```python
from build123d import *

# Parameters (mm, degrees)
SKETCH1_W             = 66.675
SKETCH1_H             = 234.95
BOSS_EXTRUDE1_DEPTH   = 3.175
SKETCH3_W             = 12.7
SKETCH3_H             = 3.175
BOSS_EXTRUDE2_DEPTH   = 3.175
CUT_EXTRUDE1_DEPTH    = 126.211389383
FILLET1_R             = 0.508
F_6_32_TAPPED_HOLE1_D = 2.7051


with BuildPart() as part:
    # Sketch1 → Boss-Extrude1 (new body)
    with BuildSketch(Plane(origin=(0, 0, 0), x_dir=(1, 0, 0), z_dir=(0, 1, 0))):
        Rectangle(SKETCH1_W, SKETCH1_H)
    extrude(amount=BOSS_EXTRUDE1_DEPTH)

    # Sketch3 → Boss-Extrude2 (add)
    with BuildSketch(Plane(origin=(0, 3.175, 0), x_dir=(1, 0, 0), z_dir=(0, 1, 0))):
        with Locations((-19.05, -119.0625)):
            Rectangle(SKETCH3_W, SKETCH3_H)
        with Locations((19.05, -119.0625)):
            Rectangle(SKETCH3_W, SKETCH3_H)
        with Locations((19.05, 119.0625)):
            Rectangle(SKETCH3_W, SKETCH3_H)
        with Locations((-19.05, 119.0625)):
            Rectangle(SKETCH3_W, SKETCH3_H)
    extrude(amount=-BOSS_EXTRUDE2_DEPTH)

    # Sketch4 → Cut-Extrude1 (cut, through all)
    with BuildSketch(Plane(origin=(0, 3.175, 0), x_dir=(1, 0, 0), z_dir=(0, 1, 0))):
        with BuildLine():
            Line((-12.7, 111.125), (12.7, 111.125))
            ThreePointArc((12.7, 111.125), (19.05, 104.775), (12.7, 98.425))
            Line((12.7, 98.425), (-12.7, 98.425))
            ThreePointArc((-12.7, 98.425), (-19.05, 104.775), (-12.7, 111.125))
        make_face()
    extrude(amount=-CUT_EXTRUDE1_DEPTH, mode=Mode.SUBTRACT)

    # Fillet1
    fillet1_edges = [part.edges().sort_by_distance(p)[0] for p in [
        (25.4, 1.5875, 117.475),
        (12.7, 1.5875, 117.475),
        (-12.7, 1.5875, 117.475),
        (-25.4, 1.5875, 117.475),
        (25.4, 1.5875, -117.475),
        (-12.7, 1.5875, -117.475),
        (-25.4, 1.5875, -117.475),
        (12.7, 1.5875, -117.475),
    ]]
    fillet(fillet1_edges, radius=FILLET1_R)

    # #6-32 Tapped Hole1 (through all)
    with Locations(Plane(origin=(-15.15, 3.175, -79.195), x_dir=(0, 0, 1), z_dir=(0, 1, 0))):
        with Locations((0, 0), (22.86, -0.18), (154.94, 0), (0, 30.3), (22.86, 30.48), (154.94, 30.3)):
            Hole(F_6_32_TAPPED_HOLE1_D / 2)


solid = part.part
```
Check sheet for the modelled part. Datum: model origin and axes. Units: mm. Give positions to 0.01 mm unless a question says otherwise; leave off trailing zeros. Loops run counter-clockwise (first coordinate to the right, second up) from the corner with the lowest first, then second, coordinate; pieces in that order, holes last. Notation, with made-up numbers: (7.5, 74.5) - (11.5, 74.5) arc R31 cw to (11.5, 99.5) - close; hole circle Ø5 at (-12.5, 39). An arc over 180 degrees is marked (long way). One line per question, with ' | ' between items. Start each with the question number.
1. Gauge pin test, flat ends, axial feed: pin 1 Ø0.8 at (y, z) = (1.5, 119.5) entering from +X; pin 2 Ø2 at (x, z) = (15.15, 75.745) entering from -Y; pin 3 Ø1.3 at (y, z) = (2, -119.5) entering from -X; pin 4 Ø1.6 at (x, y) = (-29.5, 1) entering from -Z (3 decimals). Record the tip position at first contact, or that the pin passes through.
2. Cross-section at B-B, the plane y = 2.3. Give the number of separate pieces and of enclosed holes in the cut face, plus the area to 3 significant figures.
3. Draft check along X on faces 1 (the flat face through (0, 3.175, -2)), 2 (the cylindrical face through (-19.05, 1.61, -104.64)), 3 (the cylindrical face through (19.05, 1.61, -104.91)). Enter one of: released by +X, released by -X, zero draft, split by the parting line, or undercut.
4. Cross-section at A-A, the plane x = -3. Enter the section's corners in (y, z) (3 decimals).
5. Material ranges on line 1 along Z through (x, y) = (-8, 0.25) (3 decimals); line 2 along Z through (x, y) = (-14.5, 1.85); line 3 along Z through (x, y) = (28, 0.7) (3 decimals), recorded low to high. Write a range as [from, to].
Check result:
1) pin 1: stops at x = 25.4 | pin 2: passes through | pin 3: stops at x = -25.4 | pin 4: stops at z = -117.475
2) separate pieces: 1 | enclosed holes: 7 | area: 15,300 mm2
3) face 1: zero draft | face 2: undercut | face 3: undercut
4) outline: (0, -117.475) - (3.175, -117.475) - (3.175, -111.125) - (0, -111.125) - close; (0, -98.425) - (3.175, -98.425) - (3.175, 117.475) - (0, 117.475) - close
5) line 1: z = [-117.475, -111.125], [-98.425, 117.475] | line 2: z = [-120.65, -110.86], [-98.69, -80.38], [-78.01, -57.4], [-55.27, 74.56], [76.93, 120.65] | line 3: z = [-117.475, 117.475]
